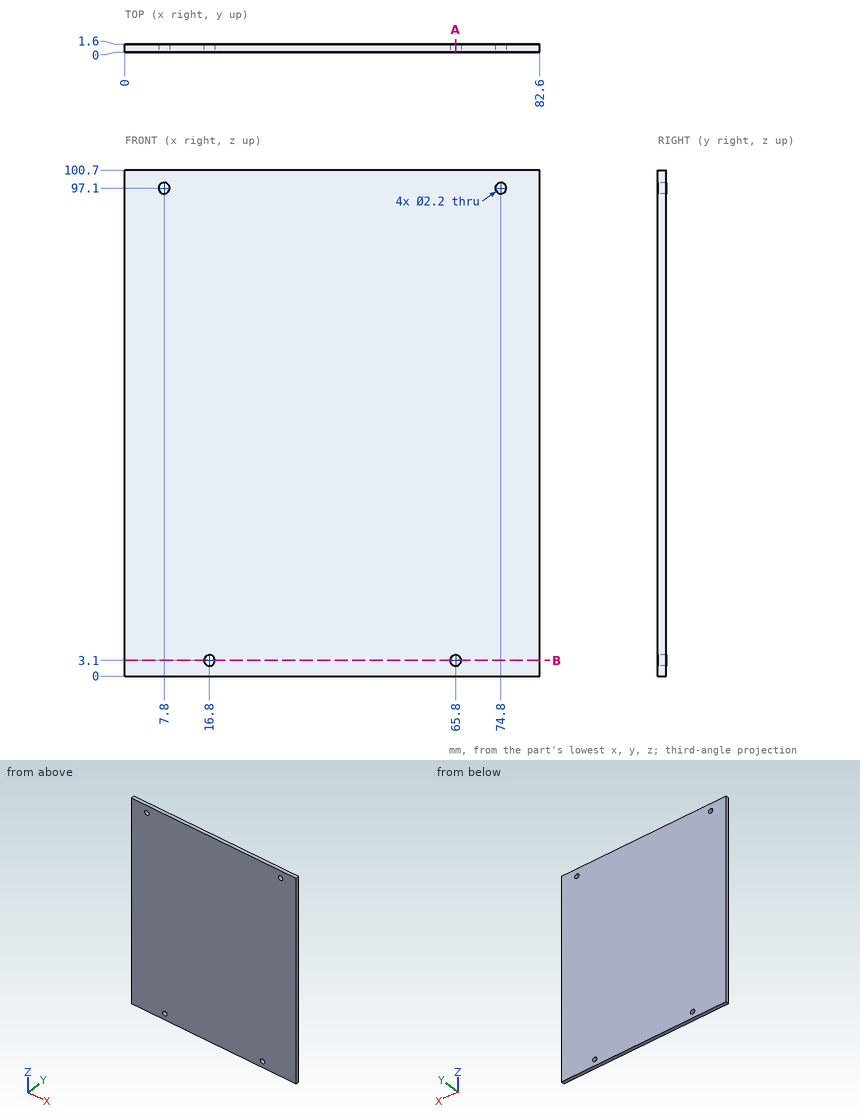
Check sheet for the drawn part. Datum: minimum x, y, z corner. Units: mm. Round coordinates to 2 decimals unless told otherwise and drop trailing zeros. Order: outer loops, then holes, each group sorted by start corner. A loop starts at its lowest first (then second) coordinate and runs counter-clockwise, first axis right, second up. Notation, with made-up numbers: (21, 56.5) -> (71, 56.5) arc R22 ccw to (71, 76.5) -> close; hole circle Ø10 at (-34, -16). An arc over 180 degrees is marked (long way). Put each result on its own line as item: value.
1) Section check A-A (x = 65.8). Record the cut outline in (y, z), then the cut area to 3 significant figures.
Final values:
outline: (0, 0) -> (1.6, 0) -> (1.6, 2) -> (0, 2) -> close; (0, 4.2) -> (1.6, 4.2) -> (1.6, 100.7) -> (0, 100.7) -> close
area: 158 mm^2
2) Material ranges on line 1 (Z direction, x = 17, y = 1.55); line 2 (Z direction, x = 7.8, y = 0.55), recorded low to high.
Final values:
line 1: z = 0 to 2.02, 4.18 to 100.7
line 2: z = 0 to 96, 98.2 to 100.7
3) Section check B-B (z = 3.1). Record the cut outline in (x, y), then the cut area to 3 significant figures.
Final values:
outline: (0, 0) -> (15.7, 0) -> (15.7, 1.6) -> (0, 1.6) -> close; (17.9, 0) -> (64.7, 0) -> (64.7, 1.6) -> (17.9, 1.6) -> close; (66.9, 0) -> (82.6, 0) -> (82.6, 1.6) -> (66.9, 1.6) -> close
area: 125 mm^2
